Model file for the job. Use its own axes, mm. Face numbers are marked on the shaded views. Give positions to 0.01 mm unless a question says otherwise; leave off trailing zeros. Loops run counter-clockwise (first coordinate to the right, second up) from the corner with the lowest first, then second, coordinate; pieces in that order, holes last. Notation, with made-up numbers: (12.25, 39) - (22.25, 39) arc R29 cw to (22.25, 77) - close; hole circle Ø7 at (17.5, 79.5). An arc over 180 degrees is marked (long way). Answer as CSV lines item,"result". Start each with the question number.
Item 1: Saw through at D-D on y = 31. Give the cut face in (x, z).
Item 2: Saw through at A-A on y = 87.5. Give the cut face in (x, z), plus the area to 3 significant figures.
Item 3: Pin check, flat tips, straight feed: pin 1 (0.8 mm diameter, centred on y = 63, z = 9.5, fed in from +X); pin 2 (1 mm diameter, centred on x = 22, y = 61, fed in from -Z); pin 3 (2 mm diameter, centred on x = 27.5, z = 2, fed in from -Y); pin 4 (0.5 mm diameter, centred on x = 35, z = 9.5, fed in from +Y). Stop position of each tip, or through.
Item 4: Pull direction Y, two halves, no side cores. Call the marked faces 1 and 2: pulls with the +Y half, pulls with the -Y half, needs draft (parallel to the pull), parting line crosses it, or undercut.
Item 5: Saw through at B-B on z = 1.75. Give the cut face in (x, y), plus the area to 3 significant figures.
Item 6: Drill centre lines: L1, parallel to Y at x = 35, z = 9.6; L2, parallel to Y at x = 35, z = 9.5; L3, parallel to X at y = 96, z = 4. Where is each one in solid material? Low to high. Write a range as from..to.
Item 7: Saw through at C-C on x = 35. Give the cut face in (y, z), plus the area to 3 significant figures.
from build123d import *

# Parameters (mm, degrees)
SKICA1_W                 = 70
SKICA1_H                 = 115
VYSUNOUT1_DEPTH          = 10
ZKOSIT1_SIZE             = 4
SKO_EPINA1_T             = -1
SKICA3_R                 = 2
SKICA3_W                 = 10
SKICA3_H                 = 25
ODEBRAT_VYSUNUT_M1_DEPTH = 11


with BuildPart() as part:
    # Skica1 → Vysunout1 (new body)
    with BuildSketch(Plane.XY):
        with Locations((35, 57.5)):
            Rectangle(SKICA1_W, SKICA1_H)
    extrude(amount=VYSUNOUT1_DEPTH)

    # Zkosit1
    zkosit1_edges = [part.edges().sort_by_distance(p)[0] for p in [
        (70, 57.5, 10),
        (35, 115, 10),
        (0, 57.5, 10),
        (35, 0, 10),
    ]]
    chamfer(zkosit1_edges, length=ZKOSIT1_SIZE)

    # Skořepina1
    sko_epina1_openings = [part.faces().sort_by_distance(p)[0] for p in [
        (35, 57.5, 0),
    ]]
    offset(amount=SKO_EPINA1_T, openings=sko_epina1_openings, kind=Kind.INTERSECTION)

    # Skica3 → Odebrat vysunutím1 (cut, through all)
    with BuildSketch(Plane.XY.offset(10)):
        with Locations((35, 87.5)):
            Circle(SKICA3_R)
        with Locations((35, 27.5)):
            Circle(SKICA3_R)
        with Locations((35, 57.5)):
            Rectangle(SKICA3_W, SKICA3_H)
    extrude(amount=-ODEBRAT_VYSUNUT_M1_DEPTH, mode=Mode.SUBTRACT)


solid = part.part
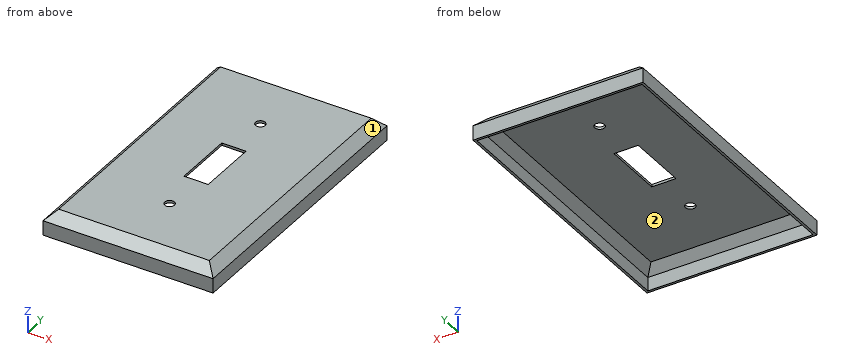
Responses:
1,outline,"(0, 0) - (1, 0) - (1, 5.59) - (4.41, 9) - (65.59, 9) - (69, 5.59) - (69, 0) - (70, 0) - (70, 6) - (66, 10) - (4, 10) - (0, 6) - close"
2,outline,"(0, 0) - (1, 0) - (1, 5.59) - (4.41, 9) - (33, 9) - (33, 10) - (4, 10) - (0, 6) - close; (37, 9) - (65.59, 9) - (69, 5.59) - (69, 0) - (70, 0) - (70, 6) - (66, 10) - (37, 10) - close"
2,area,"79.7 mm2"
3,pin 1,"x = 66.9"
3,pin 2,"z = 9"
3,pin 3,"y = 0"
3,pin 4,"y = 111.75"
4,face 1,"needs draft"
4,face 2,"undercut"
5,outline,"(0, 0) - (70, 0) - (70, 115) - (0, 115) - close; hole (1, 1) - (69, 1) - (69, 114) - (1, 114) - close"
5,area,"366 mm2"
6,L1,"3.6..25.5, 29.5..45, 70..85.5, 89.5..111.4"
6,L2,"3.5..25.5, 29.5..45, 70..85.5, 89.5..111.5"
6,L3,"0..1, 69..70"
7,outline,"(0, 0) - (1, 0) - (1, 5.59) - (4.41, 9) - (25.5, 9) - (25.5, 10) - (4, 10) - (0, 6) - close; (29.5, 9) - (45, 9) - (45, 10) - (29.5, 10) - close; (70, 9) - (85.5, 9) - (85.5, 10) - (70, 10) - close; (89.5, 9) - (110.59, 9) - (114, 5.59) - (114, 0) - (115, 0) - (115, 6) - (111, 10) - (89.5, 10) - close"
7,area,"95.7 mm2"
